```python
from build123d import *

# Parameters (mm, degrees)
F0_R            = 16.8606013276
F1_DEPTH        = 3.175
F3_DEPTH        = 3.175
F3_COPIES_COUNT = 34


# Not quite as in the source:
# - a pattern or mirror of a feature is missing from the dataset's text; its kind, count and spacing are read off the source's solid
# - a feature names something its author has since deleted; it is built from what else it names


with BuildPart() as f1:
    # F0 (on Top) → F1 (new body)
    with BuildSketch(Plane.XY):
        Circle(F0_R)
        with BuildLine():
            ThreePointArc((3.0120209, 0.8762828927), (0, -3.1369), (-3.0120209, 0.8762828927))
            Line((-3.0120209, 0.8762828927), (3.0120209, 0.8762828927))
        make_face(mode=Mode.SUBTRACT)
    extrude(amount=F1_DEPTH)

    # F2 (on face) → F3 (cut, through all)
    with BuildSketch(Plane.XY.offset(3.175)):
        with BuildLine():
            Line((0.2750051008, 14.882965874), (1.0776094804, 16.8261295293))
            ThreePointArc((1.0776094804, 16.8261295293), (0, 16.8606013276), (-1.0776094804, 16.8261295293))
            Line((-1.0776094804, 16.8261295293), (-0.2750051008, 14.882965874))
            ThreePointArc((-0.2750051008, 14.882965874), (0, 14.6990139664), (0.2750051008, 14.882965874))
        make_face()
    f3 = extrude(amount=-F3_DEPTH, mode=Mode.SUBTRACT)

    # F3_copies: F3 ×34 about axis
    f3_copies_axis = Axis((0, 0, 0), (0, 0, 1))
    for i in range(1, F3_COPIES_COUNT):
        add(f3.rotate(f3_copies_axis, i * 360 / F3_COPIES_COUNT), mode=Mode.SUBTRACT)


solid = f1.part
```
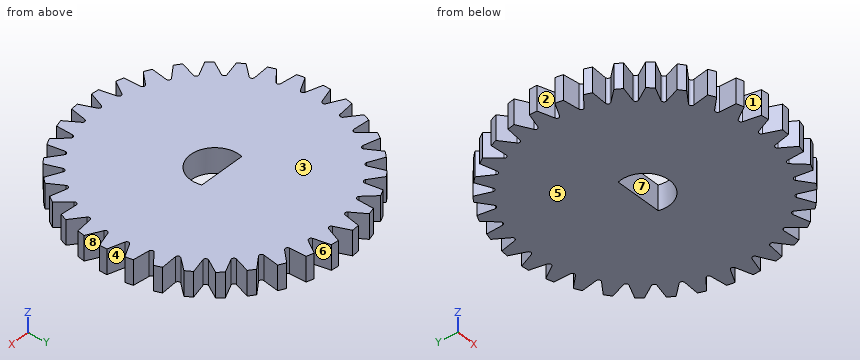
Model file for the job. Use its own axes, mm. Face numbers are marked on the shaded views. A direction names the side the tool comes from. Round coordinates to 2 decimals unless told otherwise and drop trailing zeros. Order: outer loops, then holes, each group sorted by start corner. A loop starts at its lowest first (then second) coordinate and runs counter-clockwise, first axis right, second up. Notation, with made-up numbers: (-5.5, 4) -> (24.5, 4) arc R17 ccw to (24.5, 27) -> close; hole circle Ø6 at (57.5, -5.5). An arc over 180 degrees is marked (long way). Use one line per item in the form item = value.
Item 1: Drill centre lines: line 1 (Y direction, x = 0, z = 1.05); line 2 (X direction, y = 0, z = 1.4); line 3 (Y direction, x = -6.5, z = 1.1). Where is each one in solid material? Low to high.
Returned:
line_1 = -14.7 to -3.14, 0.88 to 14.7
line_2 = -16.86 to -3.14, 3.14 to 16.86
line_3 = -14.69 to 14.69
Item 2: Pull direction X, two halves, no side cores. Call the marked faces 1, 2, 3 and 4: released by +X, released by -X, zero draft, split by the parting line, or undercut.
Returned:
face_1 = undercut
face_2 = released by -X
face_3 = zero draft
face_4 = released by +X
Item 3: Tool access for the marked faces 5, 6, 7 and 8: list every direction of +Z, -Z, +X, -X, +Y, -Y with a clear straight run to the whole face (end or side of a thin tool).
Returned:
face_5 = -Z, +X, -X, +Y, -Y
face_6 = +Z, -Z, +Y
face_7 = +Z, -Z
face_8 = +Z, -Z, +X
Item 4: Cut at A-A, the plane y = 0. Write the cut outline in (x, z) (3 decimals).
Returned:
outline = (-16.861, 0) -> (-3.137, 0) -> (-3.137, 3.175) -> (-16.861, 3.175) -> close; (3.137, 0) -> (16.861, 0) -> (16.861, 3.175) -> (3.137, 3.175) -> close
Item 5: Flat gauge pin, fed straight in: pin 1 Ø1.5 at (y, z) = (-11.5, 1) entering from +X. Where does the tip first touch, or does it go through?
Returned:
pin_1 = 12.78
Item 6: Cut at B-B, the plane x = -11. Write the cut outline in (y, z) (3 decimals), and give its area (3 significant figures).
Returned:
outline = (-11.176, 0) -> (11.176, 0) -> (11.176, 3.175) -> (-11.176, 3.175) -> close
area = 71.0 mm^2
